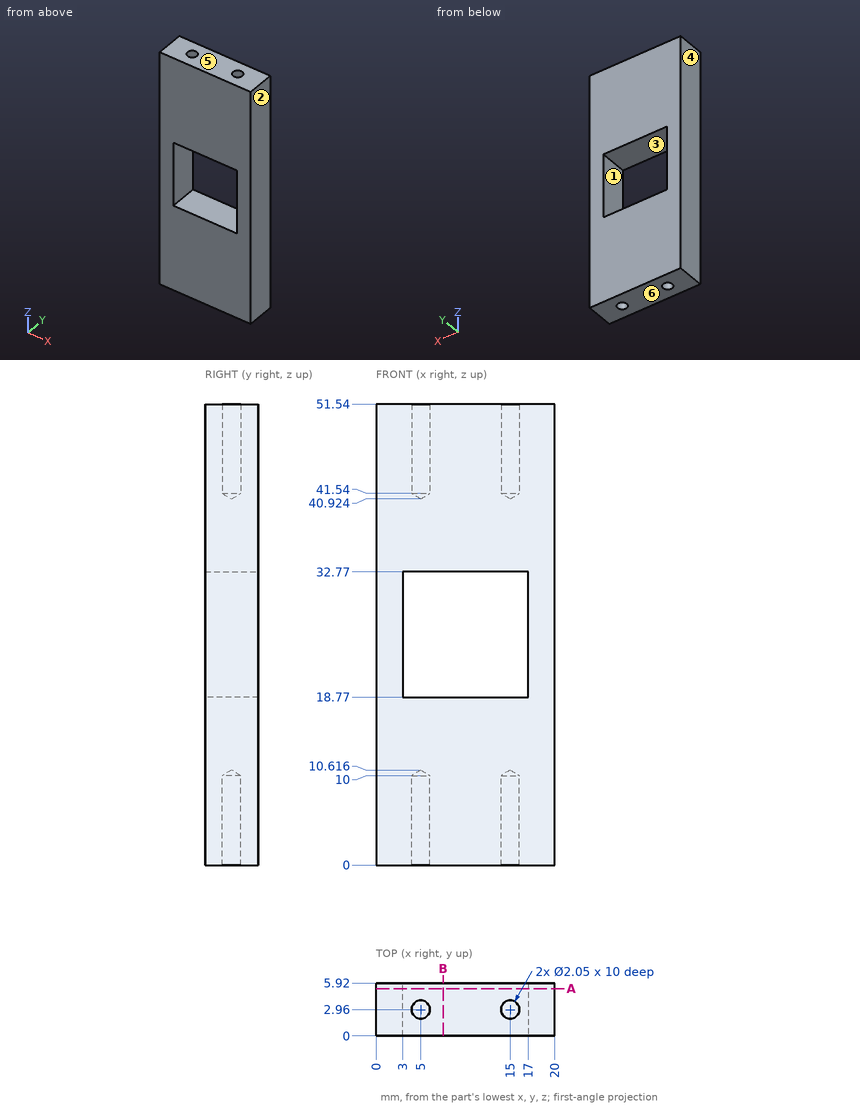
Answer from the drawing. Dimensions are ordinates in mm from the lowest x, y and z of the part. A direction names the side the tool comes from. Round coordinates to 2 decimals unless told otherwise and drop trailing zeros. Loops run counter-clockwise (first coordinate to the right, second up) from the corner with the lowest first, then second, coordinate; pieces in that order, holes last.
(1) The mould has two halves that part along Z. Classify the marked faces 3, 4, 5 and 6: pulls with the +Z half, pulls with the -Z half, needs draft (parallel to the pull), parting line crosses it, or undercut.
Computed values:
face 3: undercut
face 4: needs draft
face 5: pulls with the +Z half
face 6: pulls with the -Z half
(2) For the marked faces 1 and 2, determine the directions among +Z, -Z, +X, -X, +Y, -Y from which every point of the face is accessible in a straight line to the end or side of a thin tool.
Computed values:
face 1: +Y, -Y
face 2: +Z, -Z, +X, +Y, -Y
(3) Find the intervals of material crossed by L1, parallel to X at y = 2.96, z = 47.5 (3 decimals); L2, parallel to Z at x = 10, y = 1.35; L3, parallel to X at y = 5.1, z = 24.5, in increasing order.
Computed values:
L1: x = 0 to 3.975, 6.025 to 13.975, 16.025 to 20
L2: z = 0 to 18.77, 32.77 to 51.54
L3: x = 0 to 3, 17 to 20
(4) The part is cut by section B-B, the plane x = 7.5. Give the vertices of the cut face in (y, z).
Computed values:
outline: (0, 0) - (5.92, 0) - (5.92, 18.77) - (0, 18.77) - close; (0, 32.77) - (5.92, 32.77) - (5.92, 51.54) - (0, 51.54) - close
(5) The part is cut by section A-A, the plane y = 5.3. Give the vertices of the cut face in (x, z), and give its area (3 significant figures).
Computed values:
outline: (0, 0) - (20, 0) - (20, 51.54) - (0, 51.54) - close; hole (3, 18.77) - (17, 18.77) - (17, 32.77) - (3, 32.77) - close
area: 835 mm2
(6) Each of these flat-tipped pins is pushed along its axis until it touches: P1, Ø3, axis at x = 6, z = 13, coming from the -Y side; P2, Ø1.8, axis at x = 15, y = 2.96, coming from the +Z side (3 decimals); P3, Ø1.2, axis at x = 5, y = 2.96, coming from the +Z side. Where does it stop, or does it pass through?
Computed values:
P1: stops at y = 0
P2: stops at z = 41.465
P3: stops at z = 41.28
